```python
from build123d import *

# Parameters (mm, degrees)
SKETCH2_R               = 9.1186
SKETCH2_R_2             = 6.5532
BOSS_EXTRUDE1_DEPTH     = 20.6502
CUT_EXTRUDE1_DEPTH      = 1
CUT_EXTRUDE1_DEPTH_BACK = 3.175


with BuildPart() as part:
    # Sketch2 → Boss-Extrude1 (new body)
    with BuildSketch(Plane(origin=(0, 0, 0), x_dir=(1, 0, 0), z_dir=(0, 1, 0))):
        Circle(SKETCH2_R)
        Circle(SKETCH2_R_2, mode=Mode.SUBTRACT)
    extrude(amount=BOSS_EXTRUDE1_DEPTH)

    # Sketch3 → Cut-Extrude1 (cut, two sides)
    with BuildSketch(Plane(origin=(0, 20.6502, 0), x_dir=(1, 0, 0), z_dir=(0, 1, 0))) as cut_extrude1_sk:
        with BuildLine():
            ThreePointArc((-1.1938, 6.443544972), (0, 6.5532), (1.1938, 6.443544972))
            Line((1.1938, 6.443544972), (1.1938, 9.040116566))
            ThreePointArc((1.1938, 9.040116566), (0, 9.1186), (-1.1938, 9.040116566))
            Line((-1.1938, 9.040116566), (-1.1938, 6.443544972))
        make_face()
        with BuildLine():
            Line((1.1938, -9.040116566), (1.1938, -6.443544972))
            ThreePointArc((1.1938, -6.443544972), (0, -6.5532), (-1.1938, -6.443544972))
            Line((-1.1938, -6.443544972), (-1.1938, -9.040116566))
            ThreePointArc((-1.1938, -9.040116566), (0, -9.1186), (1.1938, -9.040116566))
        make_face()
    extrude(amount=CUT_EXTRUDE1_DEPTH, mode=Mode.SUBTRACT)
    extrude(cut_extrude1_sk.sketch, amount=-CUT_EXTRUDE1_DEPTH_BACK, mode=Mode.SUBTRACT)


solid = part.part
```
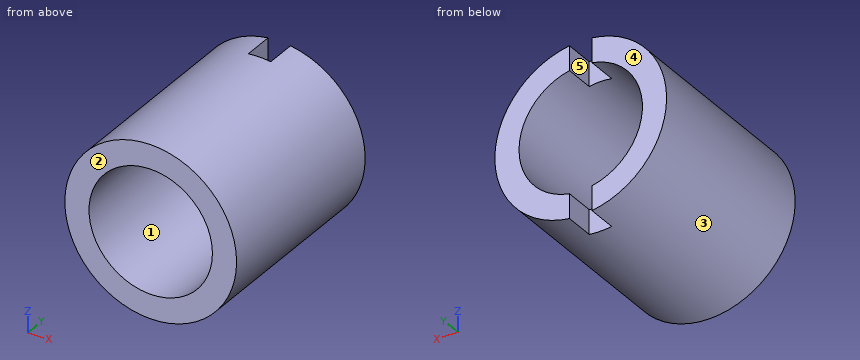
Part model, mm, in its own coordinate system. Face numbers are marked on the shaded views. A direction names the side the tool comes from. Round coordinates to 2 decimals unless told otherwise and drop trailing zeros. Loops run counter-clockwise (first coordinate to the right, second up) from the corner with the lowest first, then second, coordinate; pieces in that order, holes last.
Item 1: Drop flat-ended pins along their axis: P1, Ø3, axis at y = 19, z = -8, coming from the +X side; P2, Ø0.7, axis at x = 0, z = 7.5, coming from the +Y side; P3, Ø0.8, axis at y = 19, z = 8.5, coming from the -X side; P4, Ø4, axis at x = 0.5, z = 5, coming from the -Y side. Give the stop position or say it passes through.
Item 2: Cut at A-A, the plane x = 0. Give the cut face in (y, z).
Item 3: Drill centre lines: line 1 (Z direction, x = 0, y = 11.25); line 2 (Z direction, x = 2.75, y = 14.75). Where is each one in solid material? Low to high.
Item 4: 3-axis set-ups, long thin cutter, end or side, ignore diameter. For the marked faces 4 and 5: which of +Z, -Z, +X, -X, +Y, -Y reach the whole face in a straight line?
Item 5: Mould opens along X. For the marked faces 1, 2 and 3 say: +X half, -X half, draft (parallel to the pull), parting line (faces both ways), or undercut.
Item 6: Cut at C-C, the plane z = 7.75. Give the cut face in (x, y).
Item 7: Cut at D-D, the plane y = 6.25. Give the cut face in (x, z), then the cut area to 3 significant figures.
Item 8: Cut at B-B, the plane z = 0. Give the cut face in (x, y), then the cut area to 3 significant figures.
A:
1. P1: stops at x = 6.4
1. P2: stops at y = 17.48
1. P3: stops at x = -4.19
1. P4: stops at y = 0
2. outline: (0, -9.12) - (17.48, -9.12) - (17.48, -6.55) - (0, -6.55) - close; (0, 6.55) - (17.48, 6.55) - (17.48, 9.12) - (0, 9.12) - close
3. line 1: z = -9.12 to -6.55, 6.55 to 9.12
3. line 2: z = -8.69 to -5.95, 5.95 to 8.69
4. face 4: +Z, -Z, +X, -X, +Y
4. face 5: +Z, -Z, +Y
5. face 1: undercut
5. face 2: draft
5. face 3: parting line
6. outline: (-4.8, 0) - (4.8, 0) - (4.8, 20.65) - (1.19, 20.65) - (1.19, 17.48) - (-1.19, 17.48) - (-1.19, 20.65) - (-4.8, 20.65) - close
7. outline: circle Ø18.24 at (0, 0); hole circle Ø13.11 at (0, 0)
7. area: 126 mm2
8. outline: (-9.12, 0) - (-6.55, 0) - (-6.55, 20.65) - (-9.12, 20.65) - close; (6.55, 0) - (9.12, 0) - (9.12, 20.65) - (6.55, 20.65) - close
8. area: 106 mm2
